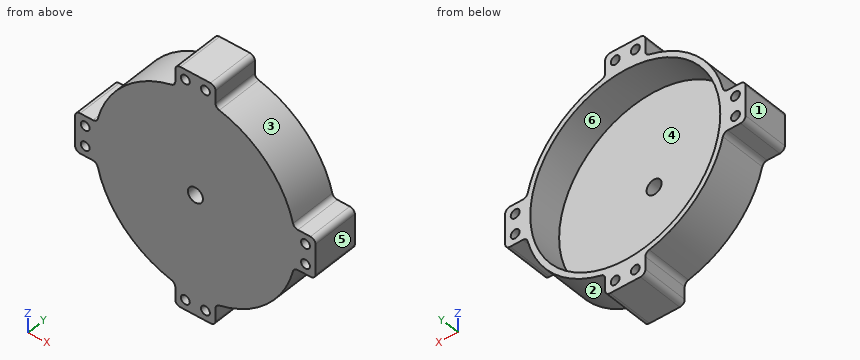
Autodesk Inventor part; units mm, degrees
ref_plane "YZ Plane" through (0, 0, 0) normal (1, 0, 0) x (0, 1, 0)
ref_plane "XZ Plane" through (0, 0, 0) normal (0, 1, 0) x (-1, 0, 0)
ref_plane "XY Plane" through (0, 0, 0) normal (0, 0, 1) x (1, 0, 0)
sketch "Sketch1" plane through (0, 0, 0) normal (0, 1, 0) x (-1, 0, 0)
  circle A0 centre (0, 0) radius 50.8
  circle A1 centre (0, 0) radius 3.81
  dimension "d0" = 101.6
  dimension "d1" = 7.62
extrude "Extrusion1" add sketch "Sketch1" along normal blind 6.35
sketch "Sketch2" plane through (0, 6.35, 0) normal (0, 1, 0) x (1, 0, 0)
  circle A0 centre (0, 0) radius 3.81
  circle A1 centre (0, 0) radius 50.8
  circle A2 centre (0, 0) radius 48.006
  dimension "d4" = 96.012
extrude "Extrusion2" add sketch "Sketch2" along normal blind 17.4498 contours A1
fillet "Fillet1" [suppressed]
sketch "Sketch3" plane through (0, 23.7998, 0) normal (0, 1, 0) x (1, 0, 0)
  circle A0 centre (0, 0) radius 48.006
  line L0 (0, 48.006) -> (10.16, 48.006)
  line L1 (10.16, 48.006) -> (10.16, 60.706)
  line L2 (10.16, 60.706) -> (0, 60.706)
  line L3 (0, 60.706) -> (0, 55.6155)
  line L4 (0, 48.006) -> (-10.16, 48.006)
  line L5 (-10.16, 48.006) -> (-10.16, 60.706)
  line L6 (-10.16, 60.706) -> (0, 60.706)
  line L7 (0, 60.706) -> (0, 55.6155)
  line L8 (-55.6768, 0) -> (-60.7568, 0)
  line L9 (-60.7568, 0) -> (-60.7568, 10.16)
  line L10 (-60.7568, 10.16) -> (-48.0568, 10.16)
  line L11 (-48.0568, 10.16) -> (-48.0568, 0)
  line L12 (-55.6768, 0) -> (-60.7568, 0)
  line L13 (-60.7568, 0) -> (-60.7568, -10.16)
  line L14 (-60.7568, -10.16) -> (-48.0568, -10.16)
  line L15 (-48.0568, -10.16) -> (-48.0568, 0)
  line L16 (0, -48.006) -> (10.16, -48.006)
  line L17 (10.16, -48.006) -> (10.16, -60.706)
  line L18 (10.16, -60.706) -> (0, -60.706)
  line L19 (0, -60.706) -> (0, -55.626)
  line L20 (0, -48.006) -> (-10.16, -48.006)
  line L21 (-10.16, -48.006) -> (-10.16, -60.706)
  line L22 (-10.16, -60.706) -> (0, -60.706)
  line L23 (0, -60.706) -> (0, -55.626)
  line L24 (48.006, 0) -> (55.626, 0)
  line L25 (60.706, 0) -> (60.706, 10.16)
  line L26 (60.706, 10.16) -> (48.006, 10.16)
  line L27 (48.006, 10.16) -> (48.006, 0)
  line L28 (48.006, 0) -> (55.626, 0)
  line L29 (60.706, 0) -> (60.706, -10.16)
  line L30 (60.706, -10.16) -> (48.006, -10.16)
  line L31 (48.006, -10.16) -> (48.006, 0)
  line L32 (5.08, -60.706) -> (5.08, -57.8739)
  line L33 (60.706, -5.08) -> (57.8739, -5.08)
  line L34 (-60.7568, -5.08) -> (-57.9247, -5.08)
  line L35 (-5.08, 60.706) -> (-5.08, 55.6155)
  circle A1 centre (-5.08, 55.6155) radius 2.2479
  circle A2 centre (5.08, 55.6155) radius 2.2479
  circle A3 centre (55.626, 5.08) radius 2.2479
  circle A4 centre (55.626, -5.08) radius 2.2479
  circle A5 centre (5.08, -55.626) radius 2.2479
  circle A6 centre (-5.08, -55.626) radius 2.2479
  circle A7 centre (-55.6768, 5.08) radius 2.2479
  circle A8 centre (-55.6768, -5.08) radius 2.2479
  line L36 (-55.6768, -5.08) -> (-55.6768, -2.8321)
  line L37 (-55.6768, 2.8321) -> (-55.6768, 5.08)
  line L38 (0, 55.6155) -> (5.08, 55.6155)
  line L39 (55.626, -5.08) -> (55.626, -2.8321)
  line L40 (55.626, 2.8321) -> (55.626, 5.08)
  line L41 (5.08, -55.626) -> (2.8321, -55.626)
  line L42 (0, -55.626) -> (-5.08, -55.626)
  point P0 (0, -60.706)
  dimension "d25" = 4.4958
  dimension "d29" = 4.4958
  dimension "d8" = 10.16
  dimension "d9" = 12.7
  dimension "d10" = 12.7
  dimension "d11" = 10.16
  dimension "d12" = 10.16
  dimension "d13" = 10.16
  dimension "d14" = 12.7
  dimension "d15" = 10.16
  dimension "d16" = 10.16
  dimension "d17" = 12.7
  dimension "d18" = 10.16
  dimension "d19" = 10.16
  dimension "d20" = 5.08
  dimension "d21" = 5.08
  dimension "d22" = 5.08
  dimension "d23" = 4.4958
  dimension "d24" = 4.4958
  dimension "d26" = 4.4958
  dimension "d27" = 4.4958
  dimension "d28" = 4.4958
  dimension "d30" = 4.4958
extrude "Extrusion3" add sketch "Sketch3" against normal up to surface (23.7998 mm away) contours L16 L17 L18 L22 L21 L20 | L4 L5 L6 L2 L1 L0 | L27 L26 L25 L29 L30 L31 | L9 L10 L11 L15 L14 L13
fillet "Fillet2" radius 2.54 16 edges at (-49.7736, 11.8999, 10.16) (-60.7568, 11.8999, 10.16) (-60.7568, 11.8999, -10.16) (-49.7736, 11.8999, -10.16) (-10.16, 11.8999, -49.7736) (-10.16, 11.8999, -60.706) (10.16, 11.8999, -60.706) (10.16, 11.8999, -49.7736) (49.7736, 11.8999, -10.16) (60.706, 11.8999, -10.16) (60.706, 11.8999, 10.16) (49.7736, 11.8999, 10.16) (10.16, 11.8999, 49.7736) (10.16, 11.8999, 60.706) (-10.16, 11.8999, 60.706) (-10.16, 11.8999, 49.7736)
properties part number "RingCase_3DPrint"
Read the model definition and answer for the solid it produces. Units are mm, in the model's axes. Face numbers are marked on the shaded views. A direction names the side the tool comes from. Coordinates: 2 decimals unless noted, no trailing zeros. Order: outer loops, then holes, each group sorted by start corner. A loop starts at its lowest first (then second) coordinate and runs counter-clockwise, first axis right, second up. Notation, with made-up numbers: (81, 22.25) -> (95, 22.25) arc R21 ccw to (95, 28.25) -> close; hole circle Ø6 at (55.5, 51.25). An arc over 180 degrees is marked (long way). Answer as a JSON object with one key per item and string values.
1) Consider line 1 along Z through (x, y) = (55.5, 22); line 2 along X through (y, z) = (15.5, -5.08); line 3 along Z through (x, y) = (-5.08, 16). Determine where each line is inside the solid, lowest interval first. Write a range as from..to.
Model answer:
{"line 1": "z = -10.16..-7.32, -2.84..2.84, 7.32..10.16", "line 2": "x = -60.76..-57.92, -53.43..-47.74, 47.74..53.38, 57.87..60.71", "line 3": "z = -60.71..-57.86, -53.37..-47.74, 47.74..53.38, 57.87..60.71"}
2) A cutting plane is placed at A-A, the plane x = 0. Determine the outline of the cut face in (y, z).
Model answer:
{"outline": "(0, -60.71) -> (23.8, -60.71) -> (23.8, -48.01) -> (6.35, -48.01) -> (6.35, -3.81) -> (0, -3.81) -> close; (0, 3.81) -> (6.35, 3.81) -> (6.35, 48.01) -> (23.8, 48.01) -> (23.8, 60.71) -> (0, 60.71) -> close"}
3) A cutting plane is placed at C-C, the plane x = -19. Determine the outline of the cut face in (y, z), plus the area to 3 significant figures.
Model answer:
{"outline": "(0, -47.11) -> (23.8, -47.11) -> (23.8, -44.09) -> (6.35, -44.09) -> (6.35, 44.09) -> (23.8, 44.09) -> (23.8, 47.11) -> (0, 47.11) -> close", "area": "704 mm²"}
4) The mould has two halves that part along Z. Classify the marked faces 1, 2, 3 and 4: released by +Z, released by -Z, zero draft, split by the parting line, or undercut.
Model answer:
{"face 1": "zero draft", "face 2": "released by -Z", "face 3": "released by +Z", "face 4": "undercut"}
5) A cutting plane is placed at B-B, the plane z = 0. Determine the outline of the cut face in (x, y), plus the area to 3 significant figures.
Model answer:
{"outline": "(-60.76, 0) -> (-3.81, 0) -> (-3.81, 6.35) -> (-48.01, 6.35) -> (-48.01, 23.8) -> (-60.76, 23.8) -> close; (3.81, 0) -> (60.71, 0) -> (60.71, 23.8) -> (48.01, 23.8) -> (48.01, 6.35) -> (3.81, 6.35) -> close", "area": "1,170 mm²"}
6) A cutting plane is placed at D-D, the plane y = 1.75. State how many separate pieces and enclosed holes the cut face has, plus the area to 3 significant figures.
Model answer:
{"separate pieces": "1", "enclosed holes": "9", "area": "8,760 mm²"}
7) Each of these flat-tipped pins is pushed along its axis until it touches: pin 1 (5 mm diameter, centred on x = 54, y = 9.5, fed in from -Z); pin 2 (4.5 mm diameter, centred on x = 0, z = 0, fed in from -Y); pin 3 (7 mm diameter, centred on y = 15, z = 54.5, fed in from +X); pin 4 (1 mm diameter, centred on x = -43.5, y = 7, fed in from -Z). Where does it stop, or does it pass through?
Model answer:
{"pin 1": "stops at z = -10.18", "pin 2": "passes through", "pin 3": "stops at x = 10.29", "pin 4": "stops at z = -27.05"}
8) A tool of negligible diameter and unlimited length cuts with its end or side. For the marked faces 5 and 6, from which of +Z, -Z, +X, -X, +Y, -Y can it reach the whole face along a straight path? Write none if from no direction.
Model answer:
{"face 5": "+Z, -Z, +X, +Y, -Y", "face 6": "+Y"}
